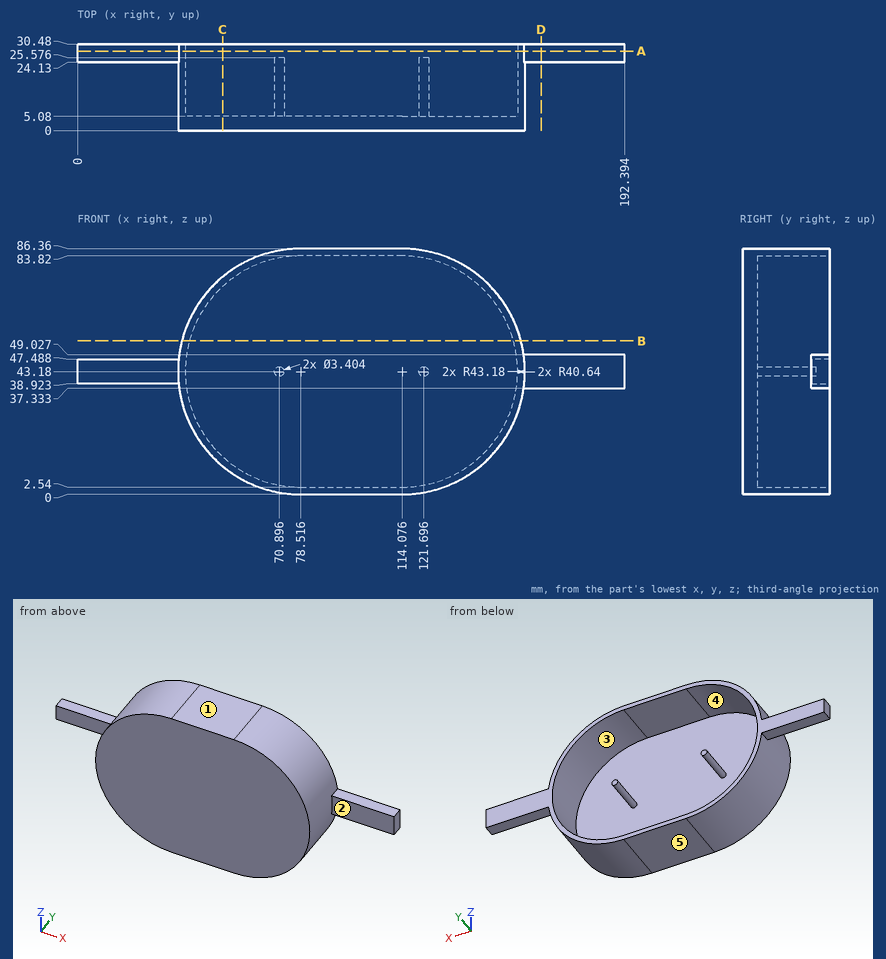
Part print with two shaded views. Sizes in mm from the minimum x, y, z corner. A direction names the side the tool comes from. Round coordinates to 2 decimals unless told otherwise and drop trailing zeros. Order: outer loops, then holes, each group sorted by start corner. A loop starts at its lowest first (then second) coordinate and runs counter-clockwise, first axis right, second up. Notation, with made-up numbers: (48.25, 77) - (80.25, 77) arc R18 ccw to (80.25, 108) - close; hole circle Ø4 at (-6.75, -30). An arc over 180 degrees is marked (long way). Answer in a Markdown table with one row per item. Add a question column.
(1) Mould opens along Z. For the marked faces 1, 2 and 3 say: +Z half, -Z half, draft (parallel to the pull), parting line (faces both ways), or undercut.
(2) Band-saw the part on B-B on z = 54. List the corners of the cut face in (x, y), and give its area (3 significant figures).
(3) 3-axis set-ups, long thin cutter, end or side, ignore diameter. For the marked faces 4 and 5: which of +Z, -Z, +X, -X, +Y, -Y reach the whole face in a straight line?
(4) Band-saw the part on A-A on y = 28. List the corners of the cut face in (x, z).
(5) Band-saw the part on D-D on x = 163. List the corners of the cut face in (y, z).
(6) Probe L1, parallel to Z at x = 82.5, y = 8; L2, parallel to Y at x = 79.5, z = 23.5; L3, parallel to X at y = 14.5, z = 70 (1 decimal). List the from-to ranges inside material, lowest first. Write a range as [from, to].
(7) Drop flat-ended pins along their axis: pin 1 Ø2.5 at (x, z) = (70.5, 43.5) entering from +Y; pin 2 Ø3 at (x, y) = (21, 27.5) entering from +Z; pin 3 Ø1 at (y, z) = (25.5, 19.5) entering from -X (1 decimal). Give the stop position or say it passes through.
(8) Band-saw the part on C-C on x = 51. List the corners of the cut face in (y, z).
Data:
| question | item | result |
|---|---|---|
| 1 | face 1 | +Z half |
| 1 | face 2 | draft |
| 1 | face 3 | undercut |
| 2 | outline | (36.71, 0) - (155.88, 0) - (155.88, 30.48) - (153.25, 30.48) - (153.25, 5.08) - (39.34, 5.08) - (39.34, 30.48) - (36.71, 30.48) - close |
| 2 | area | 739 mm^2 |
| 3 | face 4 | +Y |
| 3 | face 5 | -Z, +X, -X, +Y, -Y |
| 4 | outline | (0, 38.92) - (35.55, 38.92) arc R43.18 ccw to (78.52, 0) - (114.08, 0) arc R43.18 ccw to (156.86, 37.33) - (192.39, 37.33) - (192.39, 49.03) - (156.86, 49.03) arc R43.18 ccw to (114.08, 86.36) - (78.52, 86.36) arc R43.18 ccw to (35.55, 47.49) - (0, 47.49) - close; hole (78.52, 2.54) - (114.08, 2.54) arc R40.64 ccw to (114.08, 83.82) - (78.52, 83.82) arc R40.64 ccw to start |
| 5 | outline | (24.13, 37.33) - (30.48, 37.33) - (30.48, 49.03) - (24.13, 49.03) - close |
| 6 | L1 | z = [0, 2.54], [83.82, 86.36] |
| 6 | L2 | y = [0, 5.08] |
| 6 | L3 | x = [44.7, 48], [144.6, 147.9] |
| 7 | pin 1 | stops at y = 25.58 |
| 7 | pin 2 | stops at z = 47.49 |
| 7 | pin 3 | stops at x = 42.1 |
| 8 | outline | (0, 9.9) - (30.48, 9.9) - (30.48, 13.27) - (5.08, 13.27) - (5.08, 73.09) - (30.48, 73.09) - (30.48, 76.46) - (0, 76.46) - close |
